Model file for the job. Use its own axes, mm. Face numbers are marked on the shaded views. Give positions to 0.01 mm unless a question says otherwise; leave off trailing zeros. Write each loop counter-clockwise with the first axis right and the second up, starting at its lowest first coordinate (ties: lowest second). Pieces come first, ordered by that corner, then holes.
```python
from build123d import *

# Parameters (mm, degrees)
F0_R     = 4
F0_R_2   = 3
F1_DEPTH = 35
F3_W     = 85
F3_H     = 3.1
F4_DEPTH = 11
F5_W     = 34
F5_H     = 2
F6_DEPTH = 3.1
F9_DEPTH = 3.1
F10_R    = 8


with BuildPart() as f1:
    # F0 (on Front) → F1 (new body)
    with BuildSketch(Plane.XZ):
        Circle(F0_R)
        Circle(F0_R_2, mode=Mode.SUBTRACT)
    extrude(amount=F1_DEPTH)

    # F3 (on offset) → F4 (join)
    with BuildSketch(Plane.XZ.offset(17)):
        with Locations((7.5, 5.45)):
            Rectangle(F3_W, F3_H)
    extrude(amount=-F4_DEPTH)

    # F5 (on face) → F6 (cut)
    with BuildSketch(Plane.XY.offset(7)):
        with Locations((-18, -7)):
            Rectangle(F5_W, F5_H)
        Polygon((50, -6), (18, -6), (18, -8), align=None)
        Polygon((50, -15), (18, -17), (50, -17), align=None)
    extrude(amount=-F6_DEPTH, mode=Mode.SUBTRACT)

    # F8 (on face) → F9 (join)
    with BuildSketch(Plane(origin=(0.840745, 0, -4.768103), x_dir=(0.984808, 0, 0.173648), z_dir=(0.173648, 0, -0.984808))):
        Polygon((60.9319, 10.237065), (49.917616, 15), (49.917616, 6), (60.9319, 1.237065), align=None)
    extrude(amount=-F9_DEPTH)

    # F10
    f10_edges = [f1.edges().sort_by_distance(p)[0] for p in [
        (60.577798, -10.237065, 7.339062),
    ]]
    fillet(f10_edges, radius=F10_R)


solid = f1.part
```
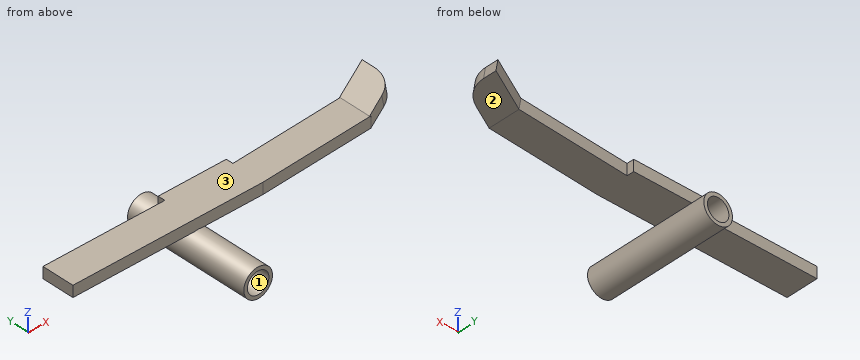
1. Probe probe 1 along Z at (x, y) = (0, -20.5); probe 2 along Z at (x, y) = (0, -10); probe 3 along Z at (x, y) = (42, -8). List the from-to ranges inside material, lowest first.
Calculated:
probe 1: z = -4 to -3, 3 to 4
probe 2: z = -4 to -3, 3 to 7
probe 3: z = 3.9 to 7
2. Slice it at D-D, the plane x = 14.5. Write the cut outline in (y, z), and give its area (3 significant figures).
Calculated:
outline: (-17, 3.9) - (-6, 3.9) - (-6, 7) - (-17, 7) - close
area: 34.1 mm2
3. Pin check, flat tips, straight feed: P1, Ø3, axis at x = 49.5, z = 4.5, coming from the +Y side; P2, Ø1, axis at y = -28.5, z = 5, coming from the +X side; P3, Ø4, axis at y = -31, z = 2, coming from the -X side; P4, Ø1, axis at y = -21.5, z = -1.5, coming from the +X side. Stop position of each tip, or through.
Calculated:
P1: stops at y = -5.52
P2: passes through
P3: stops at x = -4
P4: stops at x = 3.87
4. Slice it at B-B, the plane x = 0. Write the cut outline in (y, z).
Calculated:
outline: (-35, -4) - (0, -4) - (0, -3) - (-35, -3) - close; (-35, 3) - (0, 3) - (0, 4) - (-6, 4) - (-6, 7) - (-17, 7) - (-17, 4) - (-35, 4) - close
5. Slice it at A-A, the plane z = 0. Write the cut outline in (x, y).
Calculated:
outline: (-4, -35) - (-3, -35) - (-3, 0) - (-4, 0) - close; (3, -35) - (4, -35) - (4, 0) - (3, 0) - close
6. Slice it at C-C, the plane y = -30. Write the cut outline in (x, z), and give its area (3 significant figures).
Calculated:
outline: circle Ø8 at (0, 0); hole circle Ø6 at (0, 0)
area: 22.0 mm2
7. Pull direction Z, two halves, no side cores. Call the marked faces 1, 2 and 3: +Z half, -Z half, draft (parallel to the pull), parting line (faces both ways), or undercut.
Calculated:
face 1: undercut
face 2: -Z half
face 3: +Z half
